from build123d import *

# Parameters (mm, degrees)
F0_R          = 18
F0_R_2        = 16
F1_DEPTH      = 20.1
F0_R_3        = 22.5
F2_DEPTH      = 5
F3_W          = 5
F3_H          = 5
F4_DEPTH      = 25
F4_DEPTH_BACK = 25


with BuildPart() as f1:
    # F0 (on Top) → F1 (new body)
    with BuildSketch(Plane.XY):
        Circle(F0_R)
        Circle(F0_R_2, mode=Mode.SUBTRACT)
        Circle(F0_R_2)
    extrude(amount=F1_DEPTH)

    # F0 (on Top) → F2 (join)
    with BuildSketch(Plane.XY):
        Circle(F0_R_3)
        Circle(F0_R, mode=Mode.SUBTRACT)
    extrude(amount=F2_DEPTH)

    # F3 (on Right) → F4 (cut, two sides)
    with BuildSketch(Plane.YZ) as f4_sk:
        with Locations((0.061292029, 14.0744583309)):
            Rectangle(F3_W, F3_H)
    extrude(amount=F4_DEPTH, mode=Mode.SUBTRACT)
    extrude(f4_sk.sketch, amount=-F4_DEPTH_BACK, mode=Mode.SUBTRACT)


solid = f1.part
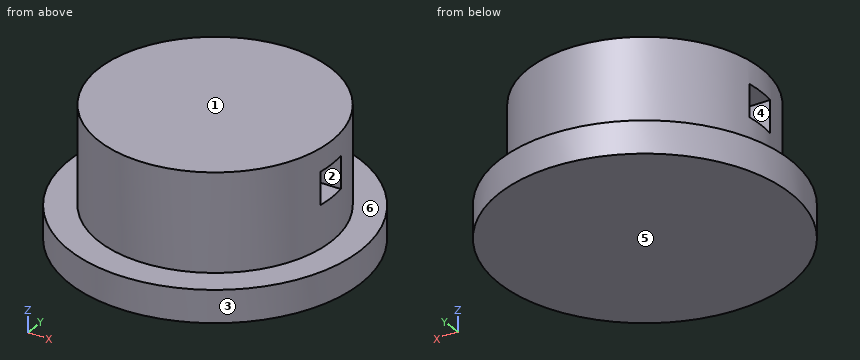
Model file for the job. Use its own axes, mm. Face numbers are marked on the shaded views. A direction names the side the tool comes from. Give positions to 0.01 mm unless a question says otherwise; leave off trailing zeros. Loops run counter-clockwise (first coordinate to the right, second up) from the corner with the lowest first, then second, coordinate; pieces in that order, holes last.
Item 1: Which spindle directions (+Z, -Z, +X, -X, +Y, -Y) get a long thin tool onto all of the face, cutting with end or side? Do the marked faces 4, 5 and 6. Say none if no direction does.
Check values:
face 4: +X, -X
face 5: -Z, +X, -X, +Y, -Y
face 6: +Z
Item 2: Slice it at A-A (x = 0). Write the cut outline in (y, z).
Check values:
outline: (-22.5, 0) - (22.5, 0) - (22.5, 5) - (18, 5) - (18, 20.1) - (-18, 20.1) - (-18, 5) - (-22.5, 5) - close; hole (-2.44, 11.57) - (2.56, 11.57) - (2.56, 16.57) - (-2.44, 16.57) - close
Item 3: Slice it at C-C (y = -10.5). Write the cut outline in (x, z), plus the area to 3 significant figures.
Check values:
outline: (-19.9, 0) - (19.9, 0) - (19.9, 5) - (14.62, 5) - (14.62, 20.1) - (-14.62, 20.1) - (-14.62, 5) - (-19.9, 5) - close
area: 641 mm2
Item 4: Mould opens along Z. For the marked faces 1, 2 and 3 say: +Z half, -Z half, draft (parallel to the pull), parting line (faces both ways), or undercut.
Check values:
face 1: +Z half
face 2: undercut
face 3: draft
Item 5: Drill centre lines: line 1 along Y through (x, z) = (-15, 15); line 2 along Z through (x, y) = (-19, -11.5); line 3 along Y through (x, z) = (0, 10.5). Where is each one in solid material? Low to high.
Check values:
line 1: y = -9.95 to -2.44, 2.56 to 9.95
line 2: z = 0 to 5
line 3: y = -18 to 18
Item 6: Slice it at B-B (z = 15.5). Write the cut outline in (x, y), plus the area to 3 significant figures.
Check values:
outline: (-17.83, -2.44) arc R18 ccw to (17.83, -2.44) - close; (-17.82, 2.56) - (17.82, 2.56) arc R18 ccw to start
area: 838 mm2
Item 7: Drop flat-ended pins along their axis: P1, Ø3, axis at x = 16, z = 9, coming from the +Y side; P2, Ø4, axis at x = -8, z = 14.5, coming from the -Y side; P3, Ø4, axis at x = -8.5, z = 14.5, coming from the +Y side. Give the stop position or say it passes through.
Check values:
P1: stops at y = 10.67
P2: stops at y = -16.97
P3: stops at y = 16.79
Item 8: Slice it at D-D (z = 9). Write the cut outline in (x, y), plus the area to 3 significant figures.
Check values:
outline: circle Ø36 at (0, 0)
area: 1,020 mm2
